For this review, take the finished solid that the model builds, in its own axes (mm). Coordinates: 2 decimals unless noted, no trailing zeros. Order: outer loops, then holes, each group sorted by start corner. A loop starts at its lowest first (then second) coordinate and runs counter-clockwise, first axis right, second up. Notation, with made-up numbers: (22.5, 43.25) -> (79.5, 43.25) arc R19 cw to (79.5, 70.25) -> close; hole circle Ø6 at (54.5, 45.25). An arc over 180 degrees is marked (long way). Answer as a JSON object with one key per item and string values. Group by question number.
1) Add section B-B, the plane y = 1.45. Write out the cut boundary in (x, z).
2) Add section A-A, the plane x = -236.5. Write out the cut boundary in (y, z) (1 decimal).
3) Add section C-C, the plane z = -217.5. Write out the cut boundary in (x, y) (3 decimals), then the cut area to 3 significant figures.
4) For pin 1 (1 mm diameter, centred on y = 1.5, z = -356.5, fed in from +X); pin 2 (1.6 mm diameter, centred on y = 2.5, z = -299, fed in from -X), all flat-tipped, find the tip position at first contact; note any pin that passes through.
5) Wall thickness on L1, parallel to Z at x = -249.5, y = 1.4; L2, parallel to X at y = 0.95, z = -198: over which ranges is each line inside the solid? List them lowest first.
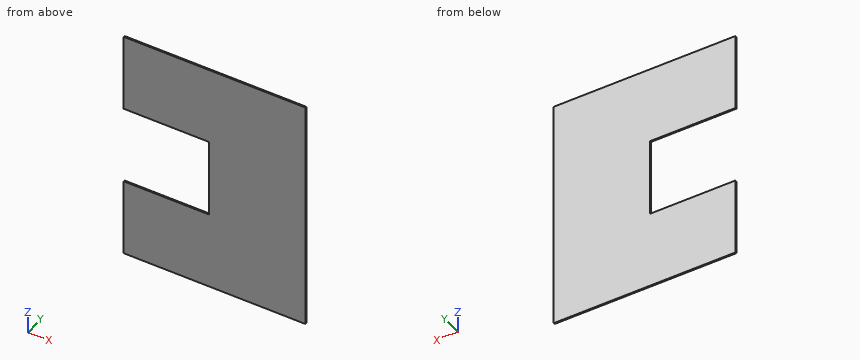
Autodesk Inventor part; units mm, degrees
ref_plane "YZ Plane" through (0, 0, 0) normal (1, 0, 0) x (0, 1, 0)
ref_plane "XZ Plane" through (0, 0, 0) normal (0, 1, 0) x (-1, 0, 0)
ref_plane "XY Plane" through (0, 0, 0) normal (0, 0, 1) x (1, 0, 0)
sketch "Sketch1" plane through (0, 0, 0) normal (0, 1, 0) x (-1, 0, 0)
  line L0 (0, 0) -> (431.8, 0)
  line L1 (431.8, 0) -> (431.8, -558.8)
  line L2 (431.8, -558.8) -> (0, -558.8)
  line L3 (0, -558.8) -> (0, 0)
  dimension "d0" = 431.8
  dimension "d1" = 558.8
extrude "Extrusion1" add sketch "Sketch1" along normal blind 3.175
sketch "Sketch3" plane through (0, 3.175, 0) normal (0, 1, 0) x (1, 0, 0)
  line L0 (0, 0) -> (0, 558.8)
  line L1 (0, 327.1063) -> (0, 139.7813)
  line L2 (-431.8, 558.8) -> (-431.8, 0)
  line L3 (-431.8, 373.0625) -> (-228.6, 373.0625)
  line L4 (-228.6, 373.0625) -> (-228.6, 185.7375)
  line L5 (-228.6, 185.7375) -> (-431.8, 185.7375)
  line L6 (-431.8, 185.7375) -> (-431.8, 373.0625)
  point P0 (-228.6, 279.4)
  point P1 (-431.8, 279.4)
  dimension "d8" = 187.325
  dimension "d9" = 203.2
extrude "Extrusion3" cut sketch "Sketch3" against normal up to surface (3.175 mm away)
properties part number "ElectricalBoard.ver1-1111-2019" material "Polycarbonate, Clear"
Output values:
{
 "1": {"outline": "(-431.8, -558.8) -> (0, -558.8) -> (0, 0) -> (-431.8, 0) -> (-431.8, -185.74) -> (-228.6, -185.74) -> (-228.6, -373.06) -> (-431.8, -373.06) -> close"},
 "2": {"outline": "(0, -558.8) -> (3.2, -558.8) -> (3.2, -373.1) -> (0, -373.1) -> close; (0, -185.7) -> (3.2, -185.7) -> (3.2, 0) -> (0, 0) -> close"},
 "3": {"outline": "(-228.6, 0) -> (0, 0) -> (0, 3.175) -> (-228.6, 3.175) -> close", "area": "726 mm²"},
 "4": {"pin 1": "stops at x = 0", "pin 2": "stops at x = -228.6"},
 "5": {"L1": "z = -558.8 to -373.06, -185.74 to 0", "L2": "x = -228.6 to 0"}
}
